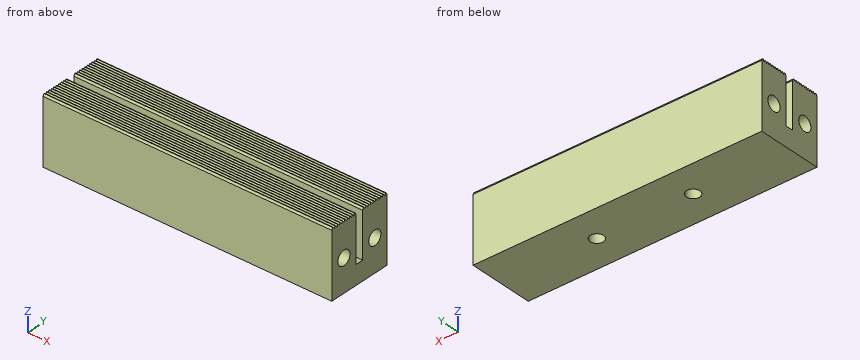
from build123d import *

# Parameters (mm, degrees)
SKETCH1_W           = 150
SKETCH1_H           = 34
BOSS_EXTRUDE1_DEPTH = 35
CUT_EXTRUDE1_DEPTH  = 160
CUT_EXTRUDE7_DEPTH  = 160
SKETCH6_W           = 0.25
SKETCH6_H           = 34
CUT_EXTRUDE8_DEPTH  = 160
SKETCH7_R           = 3.75
CUT_EXTRUDE9_DEPTH  = 160
CUT_EXTRUDE10_START = -5
SKETCH8_R           = 3.5
CUT_EXTRUDE10_DEPTH = 5


with BuildPart() as part:
    # Sketch1 → Boss-Extrude1 (new body)
    with BuildSketch(Plane.XY):
        with Locations((75, 17)):
            Rectangle(SKETCH1_W, SKETCH1_H)
    extrude(amount=BOSS_EXTRUDE1_DEPTH)

    # Sketch2 → Cut-Extrude1 (cut)
    with BuildSketch(Plane(origin=(150, 0, 0), x_dir=(0, 0, -1), z_dir=(1, 0, 0))):
        Polygon((-35, 17), (-35, 19), (-10, 19), (-10, 15), (-35, 15), align=None)
    extrude(amount=-CUT_EXTRUDE1_DEPTH, mode=Mode.SUBTRACT)

    # Sketch3 → Cut-Extrude7 (cut)
    with BuildSketch(Plane(origin=(150, 0, 0), x_dir=(0, 0, -1), z_dir=(1, 0, 0))):
        Polygon((-33.7, 19), (-35, 19.75), (-35, 18.25), align=None)
        Polygon((-33.7, 20.5), (-35, 21.25), (-35, 19.75), align=None)
        Polygon((-33.7, 22), (-35, 22.75), (-35, 21.25), align=None)
        Polygon((-33.7, 23.5), (-35, 24.25), (-35, 22.75), align=None)
        Polygon((-33.7, 25), (-35, 25.75), (-35, 24.25), align=None)
        Polygon((-33.7, 26.5), (-35, 27.25), (-35, 25.75), align=None)
        Polygon((-33.7, 28), (-35, 28.75), (-35, 27.25), align=None)
        Polygon((-33.7, 29.5), (-35, 30.25), (-35, 28.75), align=None)
        Polygon((-35, 34), (-35, 33.25), (-33.7, 34), align=None)
        Polygon((-35, 33.25), (-35, 31.75), (-33.7, 32.5), align=None)
        Polygon((-33.7, 31), (-35, 31.75), (-35, 30.25), align=None)
    cut_extrude7 = extrude(amount=-CUT_EXTRUDE7_DEPTH, mode=Mode.SUBTRACT)

    # Mirror1: Cut-Extrude7 across plane
    add(cut_extrude7.mirror(Plane.ZX.offset(17)), mode=Mode.SUBTRACT)

    # Sketch6 → Cut-Extrude8 (cut)
    with BuildSketch(Plane(origin=(150, 0, 0), x_dir=(0, 0, -1), z_dir=(1, 0, 0))):
        with Locations((-34.875, 17)):
            Rectangle(SKETCH6_W, SKETCH6_H)
    extrude(amount=-CUT_EXTRUDE8_DEPTH, mode=Mode.SUBTRACT)

    # Sketch7 → Cut-Extrude9 (cut)
    with BuildSketch(Plane(origin=(150, 0, 0), x_dir=(0, 0, -1), z_dir=(1, 0, 0))):
        with Locations((-16.85, 26.5)):
            Circle(SKETCH7_R)
        with Locations((-16.85, 7.5)):
            Circle(SKETCH7_R)
    extrude(amount=-CUT_EXTRUDE9_DEPTH, mode=Mode.SUBTRACT)

    # Sketch8 → Cut-Extrude10 (cut)
    with BuildSketch(Plane.XY.offset(10).offset(CUT_EXTRUDE10_START)):
        with Locations((100, 17)):
            Circle(SKETCH8_R)
        with Locations((50, 17)):
            Circle(SKETCH8_R)
    extrude(amount=-CUT_EXTRUDE10_DEPTH, mode=Mode.SUBTRACT)


solid = part.part
Design review of the part built by this model. Coordinates are the model's own, in mm. Coordinates: 2 decimals unless noted, no trailing zeros. Order: outer loops, then holes, each group sorted by start corner. A loop starts at its lowest first (then second) coordinate and runs counter-clockwise, first axis right, second up.
Item 1: For line 1 (Y direction, x = 85.5, z = 16.85); line 2 (Y direction, x = 73, z = 28); line 3 (Y direction, x = 100, z = 3.8), list the stretches that pass through material, from the lowest coordinate up.
Item 2: For pin 1 Ø2 at (x, y) = (99, 16.5) entering from -Z; pin 2 Ø2 at (x, y) = (85.5, 16.5) entering from +Z, all flat-tipped, find the tip position at first contact; note any pin that passes through.
Item 3: Take a section at A-A, the plane z = 16.85. Write out the cut boundary in (x, y).
Item 4: Take a section at B-B, the plane x = 50. Count the separate pieces of the cut face and the enclosed holes in it, then the cut area to 3 significant figures.
The answers:
1. line 1: y = 0 to 3.75, 11.25 to 15, 19 to 22.75, 30.25 to 34
1. line 2: y = 0 to 15, 19 to 34
1. line 3: y = 0 to 13.5, 20.5 to 34
2. pin 1: stops at z = 5
2. pin 2: stops at z = 10
3. outline: (0, 0) - (150, 0) - (150, 3.75) - (0, 3.75) - close; (0, 11.25) - (150, 11.25) - (150, 15) - (0, 15) - close; (0, 19) - (150, 19) - (150, 22.75) - (0, 22.75) - close; (0, 30.25) - (150, 30.25) - (150, 34) - (0, 34) - close
4. separate pieces: 1
4. enclosed holes: 2
4. area: 946 mm2
